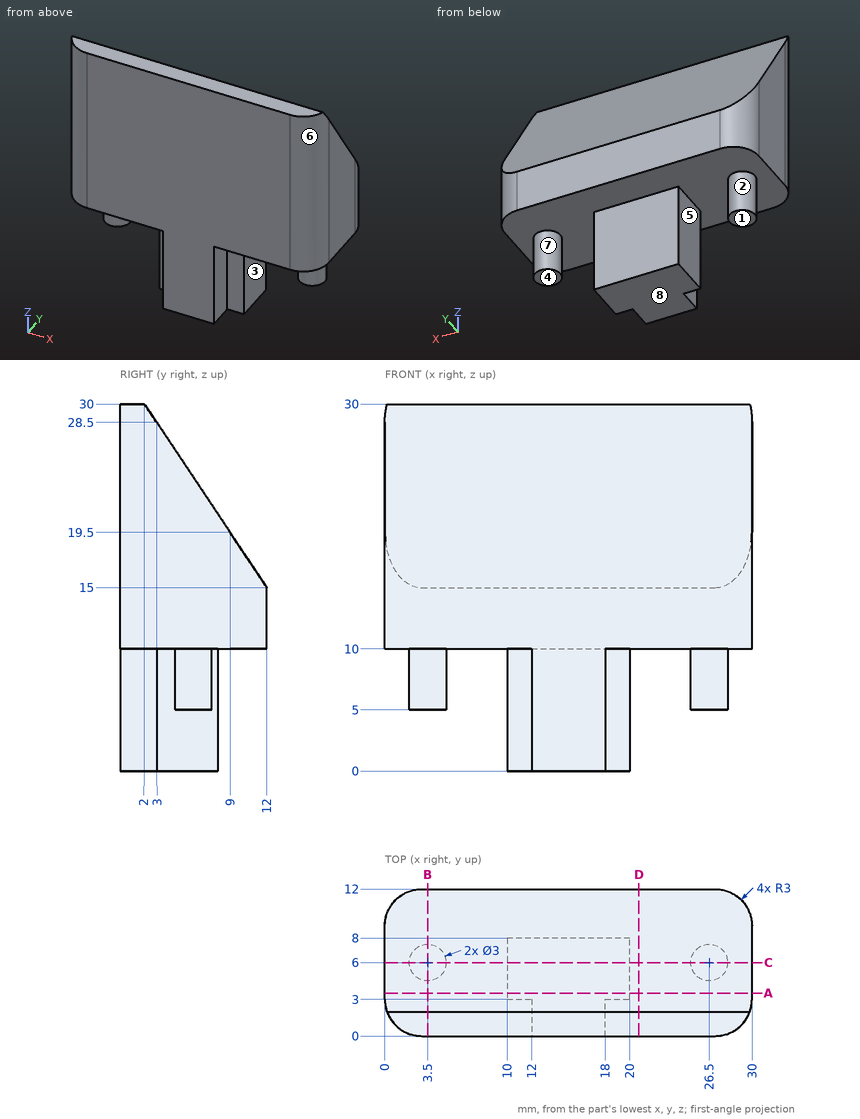
Part print with two shaded views. Sizes in mm from the minimum x, y, z corner. A direction names the side the tool comes from. Give positions to 0.01 mm unless a question says otherwise; leave off trailing zeros. Order: outer loops, then holes, each group sorted by start corner. A loop starts at its lowest first (then second) coordinate and runs counter-clockwise, first axis right, second up.
(1) Saw through at B-B, the plane x = 3.5. Give the cut face in (y, z).
(2) Mould opens along X. For the marked faces 5, 6, 7 and 8 say: released by +X, released by -X, zero draft, split by the parting line, or undercut.
(3) Drill centre lines: L1, parallel to X at y = 1, z = 7.75; L2, parallel to X at y = 3.75, z = 1.75; L3, parallel to X at y = 5.5, z = 6. Where is each one in solid material? Low to high.
(4) Saw through at A-A, the plane y = 3.5. Give the cut face in (x, z), then the cut area to 4 significant figures.
(5) Tool access for the marked faces 1, 2, 3 and 4: list every direction of +Z, -Z, +X, -X, +Y, -Y with a clear straight run to the whole face (end or side of a thin tool).
(6) Saw through at C-C, the plane y = 6. Give the cut face in (x, z).
(7) Saw through at D-D, the plane x = 20.75. Give the cut face in (y, z), then the cut area to 3 significant figures.
(8) Flat gauge pins, fed straight in: pin 1 (1 mm diameter, centred on y = 1.5, z = 17.5, fed in from -X); pin 2 (1.5 mm diameter, centred on x = 4.5, z = 20.5, fed in from +Y); pin 3 (0.9 mm diameter, centred on x = 26.5, y = 6.5, fed in from -Z). Where does each tip first touch, or does it go through?
Results found:
1. outline: (0, 10) - (4.5, 10) - (4.5, 5) - (7.5, 5) - (7.5, 10) - (12, 10) - (12, 15) - (2, 30) - (0, 30) - close
2. face 5: undercut
2. face 6: released by +X
2. face 7: undercut
2. face 8: zero draft
3. L1: x = 12 to 18
3. L2: x = 10 to 20
3. L3: x = 2.09 to 4.91, 10 to 20, 25.09 to 27.91
4. outline: (0, 10) - (10, 10) - (10, 0) - (20, 0) - (20, 10) - (30, 10) - (30, 27.75) - (0, 27.75) - close
4. area: 632.5 mm2
5. face 1: -Z, -X, +Y, -Y
5. face 2: -Z
5. face 3: -Z, +Y, -Y
5. face 4: -Z, +X, +Y, -Y
6. outline: (0, 10) - (2, 10) - (2, 5) - (5, 5) - (5, 10) - (10, 10) - (10, 0) - (20, 0) - (20, 10) - (25, 10) - (25, 5) - (28, 5) - (28, 10) - (30, 10) - (30, 24) - (0, 24) - close
7. outline: (0, 10) - (12, 10) - (12, 15) - (2, 30) - (0, 30) - close
7. area: 165 mm2
8. pin 1: stops at x = 0.17
8. pin 2: stops at y = 8.83
8. pin 3: stops at z = 5
